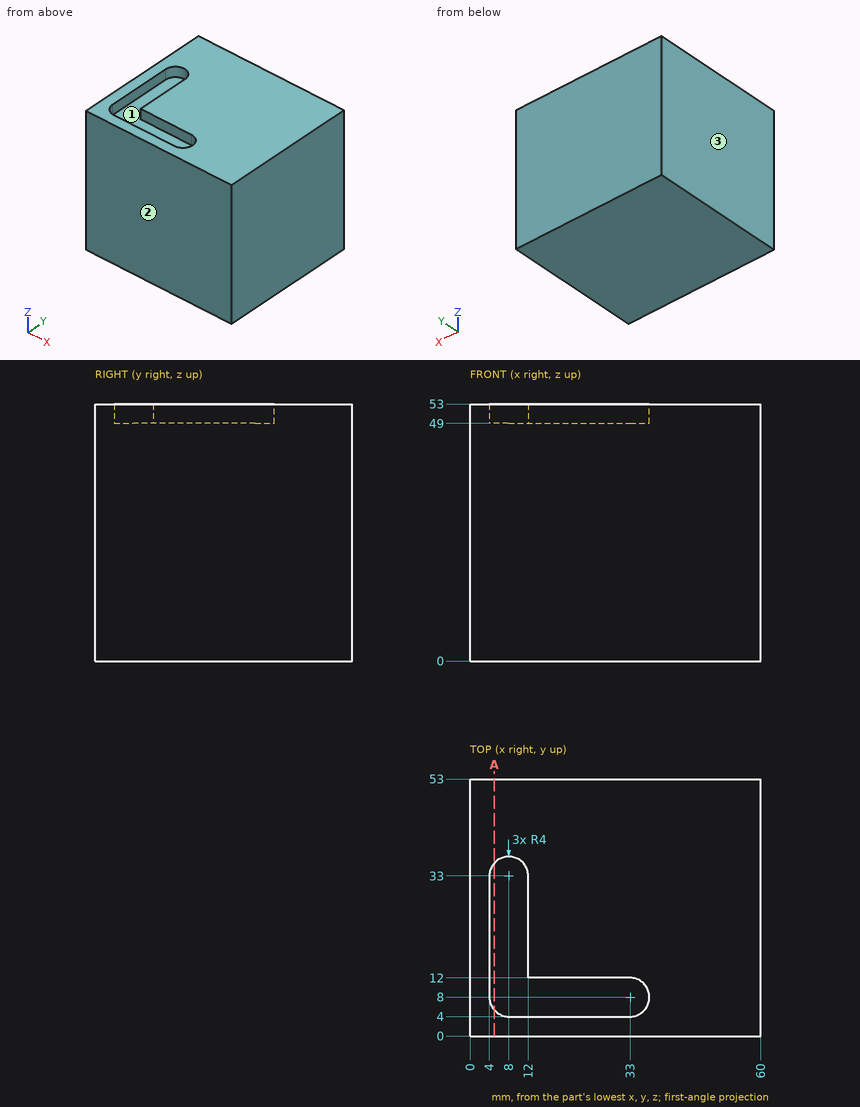
Could you check a few things on this drawing? It's one solid part, dimensions in mm from its lowest x, y, z. Give positions to 0.01 mm unless a question says otherwise; leave off trailing zeros. Write each loop counter-clockwise with the first axis right and the second up, starting at its lowest first coordinate (ties: lowest second). Pieces come first, ordered by that corner, then holes.
(1) If I drill on L1, parallel to Z at x = 12, y = 6, over which ranges is the centre line in solid material (lowest first)?
Output values:
L1: z = 0 to 49
(2) Imagine slicing it at A-A, the plane x = 5. Write out the boundary of the cut face in (y, z), and give its area (3 significant figures).
Output values:
outline: (0, 0) - (53, 0) - (53, 53) - (35.65, 53) - (35.65, 49) - (5.35, 49) - (5.35, 53) - (0, 53) - close
area: 2,690 mm2
(3) Thinking about a two-plate mould opening in Y: for the marked faces 1, 2 and 3, which applies, pulls with the +Y half, pulls with the -Y half, needs draft (parallel to the pull), parting line crosses it, or undercut?
Output values:
face 1: undercut
face 2: pulls with the -Y half
face 3: needs draft
(4) Will this pin go through, and if not, where does the flat tip stop? pin 1 (3 mm diameter, centred on x = 33.5, y = 7, fed in from +Z).
Output values:
pin 1: stops at z = 49
